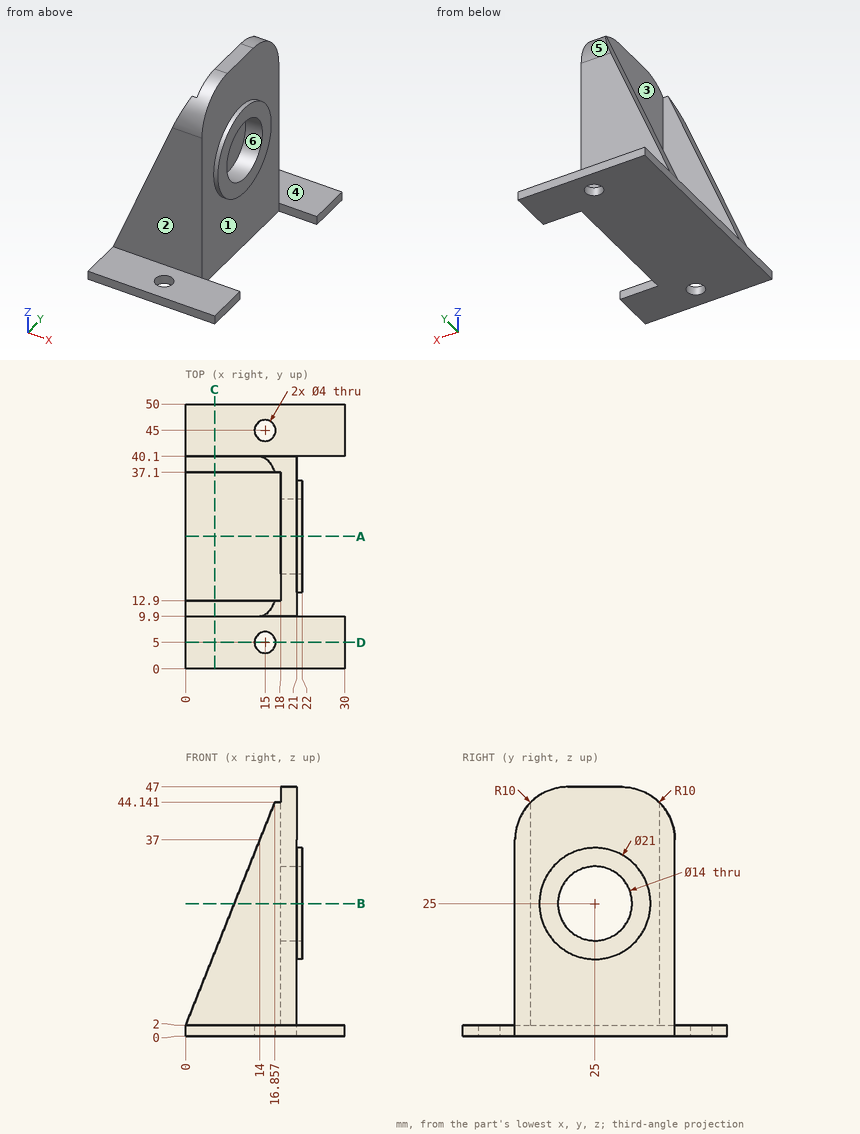
The drawing under review shows one solid part. Ordinate dimensions are in mm from its lowest x, y, z. A direction names the side the tool comes from. Coordinates: 2 decimals unless noted, no trailing zeros. Order: outer loops, then holes, each group sorted by start corner. A loop starts at its lowest first (then second) coordinate and runs counter-clockwise, first axis right, second up. Notation, with made-up numbers: (4.25, 76.5) -> (17.25, 76.5) arc R37 cw to (17.25, 113.5) -> close; hole circle Ø8 at (86.5, 37.25). An arc over 180 degrees is marked (long way). Answer as CSV lines item,"result".
Q1. Draft analysis for pull direction Y (two halves, no side actions). For the marked faces 4, 5 and 6, state which applies: released by +Y, released by -Y, zero draft, split by the parting line, or undercut.
Model answer:
face 4,"zero draft"
face 5,"released by +Y"
face 6,"undercut"
Q2. We need section D-D (y = 5). State the section outline as (x, z) points.
Model answer:
outline,"(0, 0) -> (13, 0) -> (13, 2) -> (0, 2) -> close; (17, 0) -> (30, 0) -> (30, 2) -> (17, 2) -> close"
Q3. We need section C-C (x = 5.5). State the section outline as (y, z) points.
Model answer:
outline,"(0, 0) -> (50, 0) -> (50, 2) -> (40.1, 2) -> (40.1, 15.75) -> (37.1, 15.75) -> (37.1, 2) -> (12.9, 2) -> (12.9, 15.75) -> (9.9, 15.75) -> (9.9, 2) -> (0, 2) -> close"
Q4. We need section B-B (z = 25). State the section outline as (x, y) points.
Model answer:
outline,"(9.2, 9.9) -> (21, 9.9) -> (21, 14.5) -> (22, 14.5) -> (22, 18) -> (18, 18) -> (18, 12.9) -> (9.2, 12.9) -> close; (9.2, 37.1) -> (18, 37.1) -> (18, 32) -> (22, 32) -> (22, 35.5) -> (21, 35.5) -> (21, 40.1) -> (9.2, 40.1) -> close"
Q5. We need section A-A (y = 25). State the section outline as (x, z) points.
Model answer:
outline,"(0, 0) -> (21, 0) -> (21, 14.5) -> (22, 14.5) -> (22, 18) -> (18, 18) -> (18, 2) -> (0, 2) -> close; (18, 32) -> (22, 32) -> (22, 35.5) -> (21, 35.5) -> (21, 47) -> (18, 47) -> close"
Q6. Clearance check with flat-ended pins moving along their axes: pin 1 Ø5 at (x, y) = (12, 3) entering from +Z; pin 2 Ø5 at (y, z) = (36.5, 7.5) entering from +X; pin 3 Ø8 at (x, z) = (23, 38.5) entering from -Y. State where each tip first meets the part, or that it passes through.
Model answer:
pin 1,"stops at z = 2"
pin 2,"stops at x = 21"
pin 3,"stops at y = 9.9"
Q7. For the marked faces 1, 2 and 3, list the 3-axis set-ups (+Z, -Z, +X, -X, +Y, -Y) from which the entire face can be reached by the end or side of a thin tool; tool diameter is ignored.
Model answer:
face 1,"+X"
face 2,"+Z, +X, -X, -Y"
face 3,"+Z, -X"
Q8. Wall thickness on line 1 along Y through (x, z) = (15, 1.2); line 2 along Y through (x, z) = (14.5, 5.5); line 3 along Z through (x, y) = (22, 8): over which ranges is each line inside the solid? List them lowest first. Write a range as [from, to].
Model answer:
line 1,"y = [0, 3], [7, 43], [47, 50]"
line 2,"y = [9.9, 12.9], [37.1, 40.1]"
line 3,"z = [0, 2]"
